Model file for the job. Use its own axes, mm. A direction names the side the tool comes from. Round coordinates to 2 decimals unless told otherwise and drop trailing zeros. Loops run counter-clockwise (first coordinate to the right, second up) from the corner with the lowest first, then second, coordinate; pieces in that order, holes last. Notation, with made-up numbers: (5.25, 85) - (43.25, 85) arc R24 ccw to (43.25, 114) - close; hole circle Ø11 at (57, -11). An arc over 180 degrees is marked (long way). Answer as a JSON object with one key per item and string values.
Autodesk Inventor part; units mm, degrees
ref_plane "YZ Plane" through (0, 0, 0) normal (1, 0, 0) x (0, 1, 0)
ref_plane "XZ Plane" through (0, 0, 0) normal (0, 1, 0) x (-1, 0, 0)
ref_plane "XY Plane" through (0, 0, 0) normal (0, 0, 1) x (1, 0, 0)
sketch "Skizze1" plane through (0, 0, 0) normal (0, 1, 0) x (-1, 0, 0)
  circle A0 centre (0, 0) radius 20
  dimension "d0" = 40
extrude "Extrusion1" add sketch "Skizze1" along normal blind 26
ref_plane "Arbeitsebene1" through (0, 26, 0) normal (0, 1, 0) x (1, 0, 0)
sketch "Skizze2" plane through (0, 26, 0) normal (0, 1, 0) x (1, 0, 0)
  circle A0 centre (0, 0) radius 20
  circle A1 centre (0, 0) radius 20 construction
  circle A2 centre (0, 0) radius 20 construction
  line L0 (0, 0) -> (0, 15) construction
  line L1 (0, 0) -> (0, -15) construction
  dimension "d4" = 15
  dimension "d5" = 15
hole "Bohrung1" at (0, 26, 15) at (0, 26, -15) direction (0, -1, 0) diameter 4 end through all
ref_plane "Arbeitsebene2" through (0, 0, 0) normal (0, -1, 0) x (1, 0, 0)
sketch "Skizze4" plane through (0, 0, 0) normal (0, -1, 0) x (1, 0, 0)
  point P0 (0, 0)
sketch "Skizze5" plane through (0, 0, 0) normal (0, -1, 0) x (1, 0, 0)
  line L0 (0, 0) -> (0, 20) construction
  circle A0 centre (0, 0) radius 20 construction
ref_plane "Arbeitsebene3" through (0, 0, 20) normal (0, 0, 1) x (1, 0, 0)
sketch "Skizze7" plane through (0, 0, 0) normal (0, -1, 0) x (1, 0, 0)
  circle A0 centre (0, 0) radius 5
  circle A1 centre (0, 0) radius 20
  dimension "d38" = 10
  dimension "d39" = 40
extrude "Extrusion2" cut sketch "Skizze7" against normal blind 20
sketch "Skizze8" plane through (0, 20, 0) normal (0, -1, 0) x (1, 0, 0)
  line L0 (-7.5, -25) -> (7.5, -25)
  line L1 (7.5, -25) -> (7.5, 25)
  line L2 (7.5, 25) -> (-7.5, 25)
  line L3 (-7.5, 25) -> (-7.5, -25)
  line L4 (-7.5, -25) -> (7.5, 25) construction
  line L5 (7.5, -25) -> (-7.5, 25) construction
  point P0 (0, 0)
  dimension "d42" = 15
  dimension "d43" = 50
extrude "Extrusion3" cut sketch "Skizze8" along normal through all both and the other way through all keep common part
sketch "Skizze9" plane through (0, 26, 0) normal (0, 1, 0) x (1, 0, 0)
  arc A0 (-7.5, -18.5405) -> (7.5, -18.5405) centre (0, 0) ccw
  line L0 (7.5, 18.5405) -> (-7.5, 18.5405)
  line L1 (-7.5, 18.5405) -> (-7.5, -18.5405)
  line L2 (-7.5, -18.5405) -> (7.5, -18.5405)
  line L3 (7.5, -18.5405) -> (7.5, 18.5405)
  line L4 (7.5, 18.5405) -> (-7.5, -18.5405) construction
  line L5 (-7.5, 18.5405) -> (7.5, -18.5405) construction
extrude "Extrusion4" cut sketch "Skizze9" against normal through all contours L1 L0 L3 L2 keep common part
fillet "Rundung1" radius 2 4 edges at (-7.5, 23, 18.5405) (-7.5, 23, -18.5405) (7.5, 23, 18.5405) (7.5, 23, -18.5405)
thread "Gewinde5"
thread "Gewinde6"
properties part number "spannring_achse_lager"
1) Drop flat-ended pins along their axis: P1, Ø4.5, axis at x = 0, z = 15, coming from the -Y side; P2, Ø7.5, axis at x = -3, z = 2, coming from the -Y side; P3, Ø6, axis at x = 5.5, y = 6, coming from the -Z side; P4, Ø6, axis at x = -4.5, y = 3, coming from the +Z side. Give the stop position or say it passes through.
Values follow:
{"P1": "y = 20", "P2": "y = 0", "P3": "z = -4.33", "P4": "z = 4.77"}
2) Slice it at A-A on x = 0. List the corners of the cut face in (y, z).
Values follow:
{"outline": "(0, -5) - (20, -5) - (20, -13) - (26, -13) - (26, 13) - (20, 13) - (20, 5) - (0, 5) - close; (20, -18.54) - (26, -18.54) - (26, -17) - (20, -17) - close; (20, 17) - (26, 17) - (26, 18.54) - (20, 18.54) - close"}
3) Slice it at D-D on z = 0. List the corners of the cut face in (x, y), then the cut area to 3 significant figures.
Values follow:
{"outline": "(-7.5, 20) - (-5, 20) - (-5, 0) - (5, 0) - (5, 20) - (7.5, 20) - (7.5, 26) - (-7.5, 26) - close", "area": "290 mm²"}
4) Tool access for faces 1 (the cylindrical face through (6.93, 22.96, 17.94)), 2 (the cylindrical face through (-1.08, 9.86, -4.88)): list every direction of +Z, -Z, +X, -X, +Y, -Y with a clear straight run to the whole face (end or side of a thin tool).
Values follow:
{"face 1": "+Z, +X, +Y, -Y", "face 2": "-Y"}
5) Two-plate mould, pull along Z, no slides. Class faces 3 (the flat face through (-3.4, 20, 4.4)), 4 (the cylindrical face through (6.9, 22.96, -17.97)), 5 (the cylindrical face through (1.2, 23, -16.6)): pulls with the +Z half, pulls with the -Z half, needs draft (parallel to the pull), parting line crosses it, or undercut.
Values follow:
{"face 3": "needs draft", "face 4": "pulls with the -Z half", "face 5": "undercut"}
6) Slice it at B-B on z = -15. List the corners of the cut face in (x, y).
Values follow:
{"outline": "(-7.5, 20) - (-2, 20) - (-2, 26) - (-7.5, 26) - close; (2, 20) - (7.5, 20) - (7.5, 26) - (2, 26) - close"}
7) Slice it at C-C on x = -4. List the corners of the cut face in (y, z), then the cut area to 3 significant figures.
Values follow:
{"outline": "(0, -3) - (20, -3) - (20, -18.54) - (26, -18.54) - (26, 18.54) - (20, 18.54) - (20, 3) - (0, 3) - close", "area": "342 mm²"}
8) Probe probe 1 along Z at (x, y) = (0, 24.35); probe 2 along X at (y, z) = (23.8, -15); probe 3 along Z at (x, y) = (-1.25, 21.75). List the from-to ranges inside material, lowest first.
Values follow:
{"probe 1": "-18.54 to -17, -13 to 13, 17 to 18.54", "probe 2": "-7.5 to -2, 2 to 7.5", "probe 3": "-18.54 to -16.56, -13.44 to 13.44, 16.56 to 18.54"}
